Verification items for this drawing (mm, ordinates from the low corner). Round coordinates to 2 decimals unless told otherwise and drop trailing zeros. Loops run counter-clockwise (first coordinate to the right, second up) from the corner with the lowest first, then second, coordinate; pieces in that order, holes last. Notation, with made-up numbers: (84, 1.25) - (116, 1.25) arc R31 ccw to (116, 30.25) - close; hole circle Ø8 at (9, 24). An arc over 180 degrees is marked (long way). Write item = value, one per line.
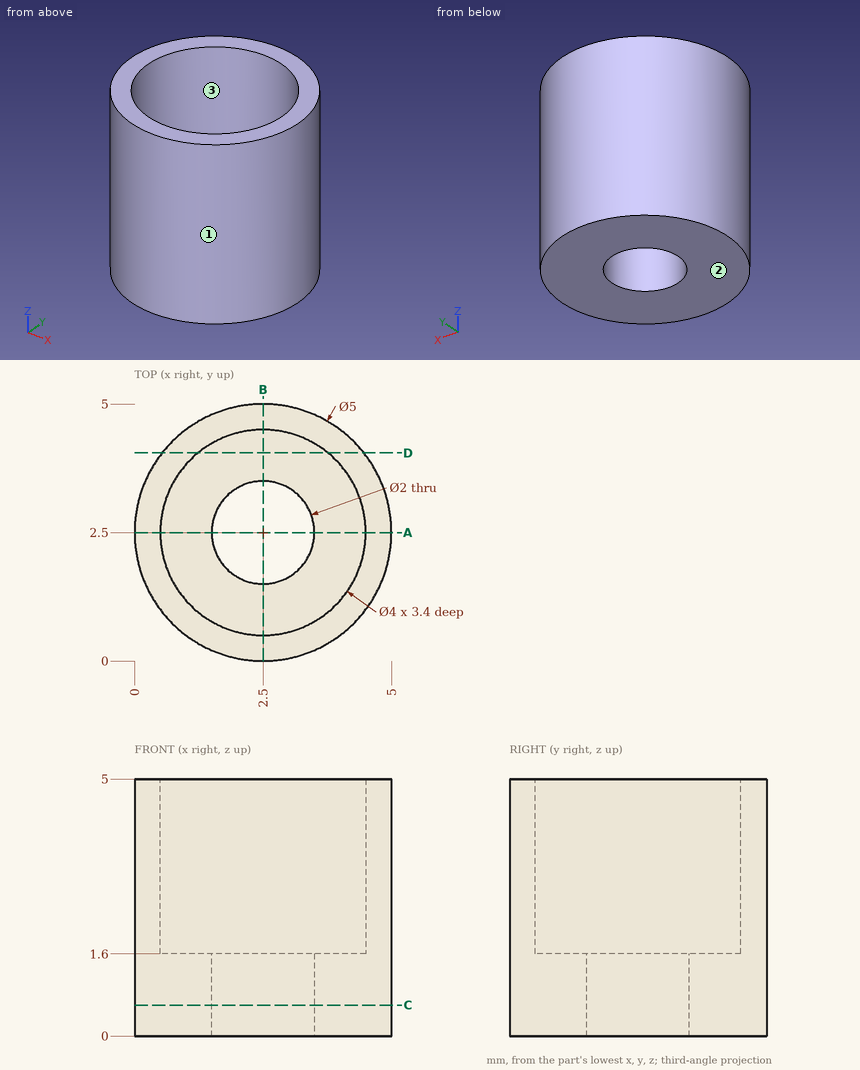
(1) Mould release check, pull along X, two halves, no side actions. Record for the marked faces 1, 2 and 3: pulls with the +X half, pulls with the -X half, needs draft (parallel to the pull), parting line crosses it, or undercut.
Answers follow:
face_1 = parting line crosses it
face_2 = needs draft
face_3 = undercut
(2) Scan lines: L1, parallel to Y at x = 2.5, z = 0.9; L2, parallel to Y at x = 2.5, z = 3.25; L3, parallel to X at y = 1.25, z = 2.85. Record each from-to range of solid material in increasing order. Write a range as [from, to].
Answers follow:
L1 = [0, 1.5], [3.5, 5]
L2 = [0, 0.5], [4.5, 5]
L3 = [0.33, 0.94], [4.06, 4.67]
(3) Section check C-C (z = 0.6). Enter the section's corners in (x, y), then the cut area to 3 significant figures.
Answers follow:
outline = circle Ø5 at (2.5, 2.5); hole circle Ø2 at (2.5, 2.5)
area = 16.5 mm²
(4) Section check D-D (y = 4.05). Enter the section's corners in (x, z), then the cut area to 3 significant figures.
Answers follow:
outline = (0.54, 0) - (4.46, 0) - (4.46, 5) - (3.76, 5) - (3.76, 1.6) - (1.24, 1.6) - (1.24, 5) - (0.54, 5) - close
area = 11.0 mm²
(5) Section check A-A (y = 2.5). Enter the section's corners in (x, z).
Answers follow:
outline = (0, 0) - (1.5, 0) - (1.5, 1.6) - (0.5, 1.6) - (0.5, 5) - (0, 5) - close; (3.5, 0) - (5, 0) - (5, 5) - (4.5, 5) - (4.5, 1.6) - (3.5, 1.6) - close
(6) Gauge pin test, flat end, axial feed: pin 1 (3 mm diameter, centred on x = 2.5, y = 2.5, fed in from +Z). Record the tip position at first contact, or that the pin passes through.
Answers follow:
pin_1 = 1.6
